from build123d import *

# Parameters (mm, degrees)
F0_R     = 15
F1_DEPTH = 3
F3_DEPTH = 3.5
F4_R     = 2


with BuildPart() as f1:
    # F0 (on Top) → F1 (new body)
    with BuildSketch(Plane.XY):
        Circle(F0_R)
    extrude(amount=F1_DEPTH)

    # F2 (on Front) → F3 (cut, symmetric)
    with BuildSketch(Plane.XZ):
        Polygon((15, 3), (-15, 3), (-15, 1.5), (15, 2.4), align=None)
    extrude(amount=F3_DEPTH, both=True, mode=Mode.SUBTRACT)

    # F4
    f4_edges = [f1.edges().sort_by_distance(p)[0] for p in [
        (-14.585952, 3.5, 2.256211),
        (14.585952, 3.5, 2.693789),
        (14.585952, -3.5, 2.693789),
        (-14.585952, -3.5, 2.256211),
    ]]
    fillet(f4_edges, radius=F4_R)


solid = f1.part
Model file for the job. Use its own axes, mm. A direction names the side the tool comes from. Give positions to 0.01 mm unless a question says otherwise; leave off trailing zeros. Order: outer loops, then holes, each group sorted by start corner. A loop starts at its lowest first (then second) coordinate and runs counter-clockwise, first axis right, second up. Notation, with made-up numbers: M 6.25,44 L 61.25,44 A32 cw 61.25,79 Z; hole C 21,86 d2. An arc over 180 degrees is marked long. Put each result on its own line as item: value. Start each with the question number.
(1) Pin check, flat tips, straight feed: pin 1 Ø1 at (x, y) = (11.5, -0.5) entering from +Z; pin 2 Ø1.5 at (y, z) = (-7.5, 2.5) entering from -X; pin 3 Ø1.5 at (x, z) = (-8, 2.5) entering from -Y; pin 4 Ø12 at (x, y) = (-7.5, 11.5) entering from -Z. Stop position of each tip, or through.
(2) Drill centre lines: L1, parallel to Y at x = -12.5, z = 1.8; L2, parallel to Y at x = -8.75, z = 2.25; L3, parallel to Z at x = 12, y = -0.5. Where is each one in solid material? Low to high. Write a range as [from, to].
(3) Band-saw the part on C-C on z = 0.8. Give the cut face in (x, y).
(4) Band-saw the part on B-B on y = -5.25. Give the cut face in (x, z).
(5) Band-saw the part on A-A on x = 0. Give the cut face in (y, z).
(6) Tool access for faces 4 (the face through (0, 8, 3)), 5 (the face through (-13.48, 4.45, 2.26)): list every direction of +Z, -Z, +X, -X, +Y, -Y with a clear straight run to the whole face (end or side of a thin tool).
(7) Band-saw the part on D-D on y = 0. Give the cut face in (x, z).
(8) Pull direction Y, two halves, no side cores. Call faces 1 (the face through (13.856, -5.745, 1.479)), 2 (the face through (0, -8, 3)), 3 (the face through (13.48, 4.45, 2.65)): released by +Y, released by -Y, zero draft, split by the parting line, or undercut.
Results below:
1. pin 1: stops at z = 2.31
1. pin 2: stops at x = -13.4
1. pin 3: stops at y = -13.13
1. pin 4: stops at z = 0
2. L1: y = [-8.29, -3.63], [3.63, 8.29]
2. L2: y = [-12.18, -3.5], [3.5, 12.18]
2. L3: z = [0, 2.31]
3. outline: C 0,0 d30
4. outline: M -14.05,0 L 14.05,0 L 14.05,2.37 L 13.76,2.36 L 13.76,3 L -13.76,3 L -13.76,1.54 L -14.05,1.53 Z
5. outline: M -15,0 L 15,0 L 15,3 L 3.5,3 L 3.5,1.95 L -3.5,1.95 L -3.5,3 L -15,3 Z
6. face 4: +Z, +X, -X, +Y, -Y
6. face 5: +Z, -X
7. outline: M -15,0 L 15,0 L 15,2.4 L -15,1.5 Z
8. face 1: split by the parting line
8. face 2: zero draft
8. face 3: undercut
